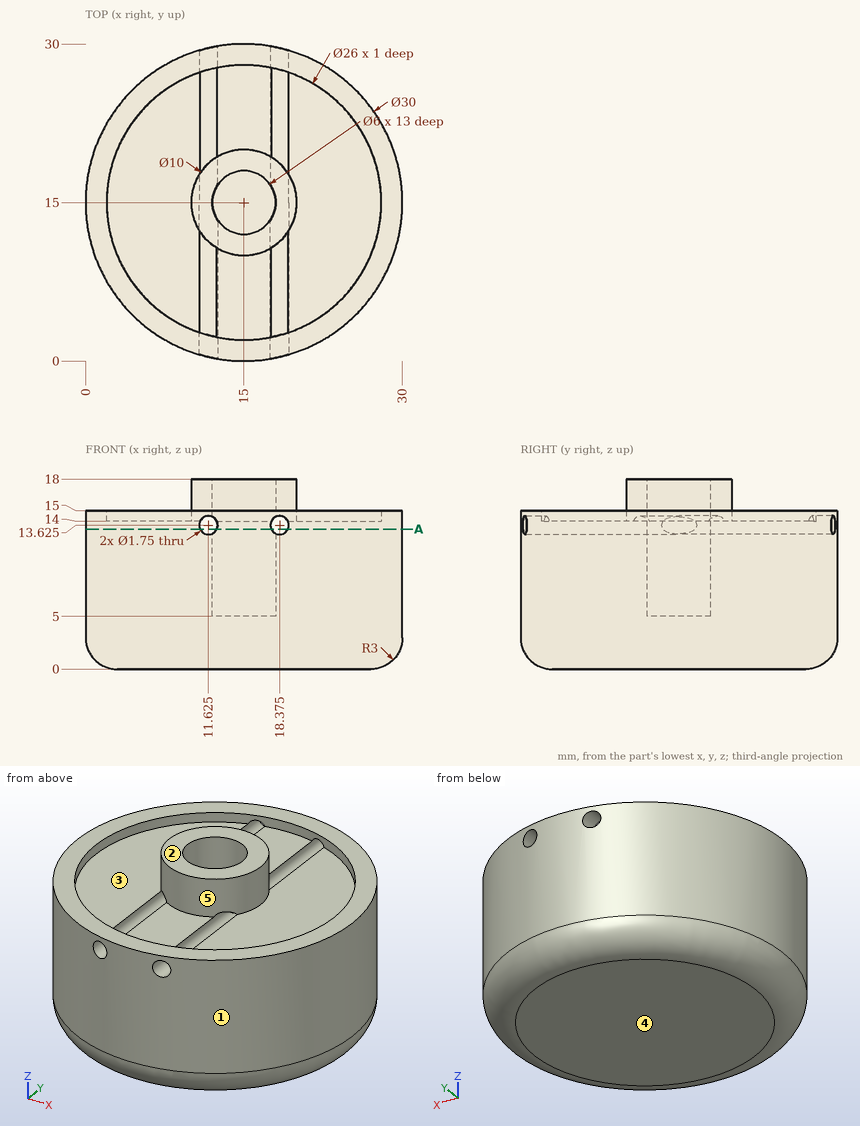
Verification items for this drawing (mm, ordinates from the low corner). A direction names the side the tool comes from. Round coordinates to 2 decimals unless told otherwise and drop trailing zeros. Write each loop counter-clockwise with the first axis right and the second up, starting at its lowest first coordinate (ties: lowest second). Pieces come first, ordered by that corner, then holes. Notation, with made-up numbers: M 36.5,51.25 L 73.5,51.25 A22 cw 73.5,84.25 Z; hole C 2.5,89 d11. An arc over 180 degrees is marked long. Write item = value, one per line. Start each with the question number.
1. Gauge pin test, flat ends, axial feed: pin 1 (12 mm diameter, centred on x = 4, y = 18, fed in from +Z); pin 2 (2 mm diameter, centred on y = 24.5, z = 15, fed in from -X); pin 3 (4.5 mm diameter, centred on x = 8, y = 10.5, fed in from +Z); pin 4 (1.4 mm diameter, centred on x = 18.375, z = 13.625, fed in from +Y). Record the tip position at first contact, or that the pin passes through.
2. Release check for a two-part mould opening along Y. For the marked faces 1, 2 and 3 record: pulls with the +Y half, pulls with the -Y half, needs draft (parallel to the pull), parting line crosses it, or undercut.
3. Tool access check on the marked faces 4 and 5. Record the directions out of +Z, -Z, +X, -X, +Y, -Y that give a thin tool (end or side, any length) a straight path to the whole face; none if there is none.
4. Scan lines: line 1 (Z direction, x = 25, y = 13.5); line 2 (Z direction, x = 16, y = 14); line 3 (Y direction, x = 6, z = 9.5). Record each from-to range of solid material in increasing order. Write a range as [from, to].
5. Section check A-A, the plane z = 13.25. Record the cut outline in (x, y), then the cut area to 3 significant figures.
Results found:
q1.pin_1 = 15
q1.pin_2 = 2.64
q1.pin_3 = 14
q1.pin_4 = through
q2.face_1 = parting line crosses it
q2.face_2 = needs draft
q2.face_3 = undercut
q3.face_4 = -Z, +X, -X, +Y, -Y
q3.face_5 = +Z
q4.line_1 = [0, 14]
q4.line_2 = [0, 5]
q4.line_3 = [3, 27]
q5.outline = M 10.83,0.59 L 10.83,29.41 A15 ccw Z; M 12.42,0.22 A15 ccw 17.58,0.22 L 17.58,13.48 A3 cw 12.42,13.48 Z; M 12.42,16.52 A3 cw 17.58,16.52 L 17.58,29.78 A15 ccw 12.42,29.78 Z; M 19.17,0.59 A15 ccw 19.17,29.41 Z
q5.area = 588 mm^2
